Read the model definition and answer for the solid it produces. Units are mm, in the model's axes. Face numbers are marked on the shaded views. A direction names the side the tool comes from. Give positions to 0.01 mm unless a question says otherwise; leave off trailing zeros. Order: outer loops, then holes, each group sorted by start corner. A loop starts at its lowest first (then second) coordinate and runs counter-clockwise, first axis right, second up.
Item 1: A cutting plane is placed at C-C (z = 2). Write down the section's boundary in (x, y), plus the area to 3 significant figures.
Item 2: Which of the six approach directions +Z, -Z, +X, -X, +Y, -Y give full straight-line access (tool end or side, diameter ignored) to the marked faces 4, 5, 6 and 7?
Item 3: A cutting plane is placed at B-B (x = 0.5). Write down the section's boundary in (y, z), plus the area to 3 significant figures.
Item 4: A cutting plane is placed at D-D (y = 2.25). Write down the section's boundary in (x, z), plus the area to 3 significant figures.
Item 5: A cutting plane is placed at A-A (y = 0.25). Write down the section's boundary in (x, z).
Item 6: The mould has two halves that part along X. Classify the marked faces 1, 2 and 3: +X half, -X half, draft (parallel to the pull), parting line (faces both ways), or undercut.
Item 7: Given pin 1 Ø3.5 at (x, y) = (0, 3) entering from +Z; pin 2 Ø0.5 at (x, z) = (-2, 0.5) entering from +Y; pin 3 Ø2 at (y, z) = (0, 2.5) entering from +X, each flat-ended and moving along its own axis, determine where each tip first touches the part or whether it passes through.
Item 8: Find the intervals of material crossed by line 1 along Z through (x, y) = (1.5, 4.5); line 2 along Y through (x, z) = (2.75, 1.1); line 3 along Y through (x, z) = (0.5, 3.6), in increasing order.
from build123d import *

# Parameters (mm, degrees)
BOSS_EXTRUDE1_DEPTH = 6
BOSS_EXTRUDE2_DEPTH = 2
CUT_EXTRUDE1_DEPTH  = 3


with BuildPart() as part:
    # Sketch2 → Boss-Extrude1 (new body)
    with BuildSketch(Plane.XY):
        with BuildLine():
            ThreePointArc((-1, 2), (4.121320344, 4.121320344), (2, -1))
            Line((2, -1), (-1, -1))
            Line((-1, -1), (-1, 2))
        make_face()
        with BuildLine():
            Line((0, 0), (0, 2))
            ThreePointArc((0, 2), (3.414213562, 3.414213562), (2, 0))
            Line((2, 0), (0, 0))
        make_face(mode=Mode.SUBTRACT)
    extrude(amount=BOSS_EXTRUDE1_DEPTH)

    # Sketch3 → Boss-Extrude2 (add)
    with BuildSketch(Plane.ZY.offset(1)):
        with BuildLine():
            Line((0, 2), (0, -1))
            Line((0, -1), (4, -1))
            ThreePointArc((4, -1), (3.121320344, 1.121320344), (1, 2))
            Line((1, 2), (0, 2))
        make_face()
    extrude(amount=BOSS_EXTRUDE2_DEPTH)

    # Sketch4 → Cut-Extrude1 (cut)
    with BuildSketch(Plane.ZY.offset(1)):
        with BuildLine():
            Line((3, 2), (4, 2))
            ThreePointArc((4, 2), (5.414213562, 1.414213562), (6, 0))
            Line((6, 0), (6, 5))
            Line((6, 5), (3, 5))
            Line((3, 5), (3, 2))
        make_face()
    extrude(amount=-CUT_EXTRUDE1_DEPTH, mode=Mode.SUBTRACT)


solid = part.part
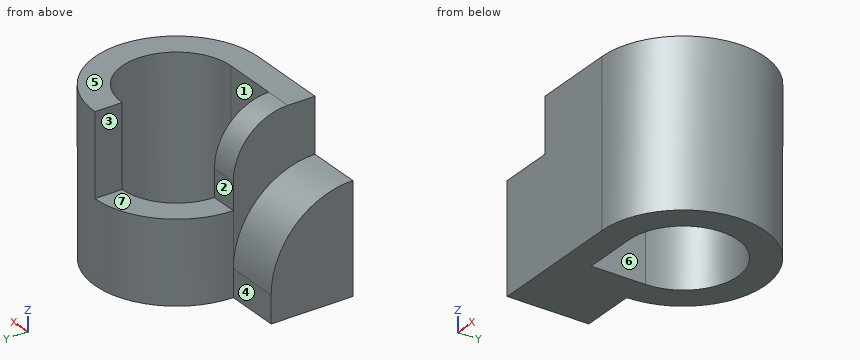
Response values:
1. outline: (-3, -1) - (2, -1) arc R3 ccw (long way) to (-1, 2) - (-1, 1.83) - (-3, 1.83) - close; hole (0, 0) - (2, 0) arc R2 ccw (long way) to (0, 2) - close
1. area: 22.4 mm2
2. face 4: +Z, -Z, -X, +Y
2. face 5: +Z, +X, -X, +Y, -Y
2. face 6: +Z, -Z
2. face 7: +Z, -X, +Y
3. outline: (-1, 0) - (0, 0) - (0, 6) - (-1, 6) - close; (3.32, 0) - (4.6, 0) - (4.6, 3) - (3.32, 3) - close
3. area: 9.83 mm2
4. outline: (-0.99, 0) - (0.02, 0) - (0.02, 3) - (-0.99, 3) - close; (3.98, 0) - (4.99, 0) - (4.99, 6) - (3.98, 6) - close
4. area: 9.05 mm2
5. outline: (-3, 0) - (0, 0) - (0, 5.98) - (-1, 5.98) - (-1, 3.73) - (-3, 3.73) - close; (2.97, 0) - (4.44, 0) - (4.44, 6) - (2.97, 6) - close
6. face 1: undercut
6. face 2: draft
6. face 3: -X half
7. pin 1: stops at z = 5.56
7. pin 2: stops at y = 2
7. pin 3: stops at x = 4.83
8. line 1: z = 0 to 3
8. line 2: y = -0.9 to 0.15, 3.85 to 4.9
8. line 3: y = -1 to 0
